Geometry check sheet. Reference: the model listing, model coordinates, mm. A direction names the side the tool comes from. Coordinates: 2 decimals unless noted, no trailing zeros. Write each loop counter-clockwise with the first axis right and the second up, starting at its lowest first coordinate (ties: lowest second). Pieces come first, ordered by that corner, then holes. Notation, with made-up numbers: (61, 69) -> (101, 69) arc R18 cw to (101, 91) -> close; hole circle Ø9 at (78, 36.25). An arc over 180 degrees is marked (long way). Answer in a Markdown table with one row per item. Add a question column.
Q1. Section check D-D, the plane x = -15. Record the boundary of the cut face in (y, z).
Q2. Section check B-B, the plane x = 53.5. Record the boundary of the cut face in (y, z), and give its area (3 significant figures).
Q3. Tool access check on faces 1 (the face through (17.734, -76, -7)), 2 (the face through (-31, -56.815, 23)), 3 (the face through (35, -32, -27.231)), 4 (the face through (-35, -14, 27.231)), 5 (the face through (-36, -42, -17.718)). Record the directions out of +Z, -Z, +X, -X, +Y, -Y that give a thin tool (end or side, any length) a straight path to the whole face; none if there is none.
Q4. Release check for a two-part mould opening along X. For faces 6 (the face through (-35, -70, 27.231)), 7 (the face through (10.484, -48.74, -9.389)), 8 (the face through (-71.588, -42, 5)) record: pulls with the +X half, pulls with the -X half, needs draft (parallel to the pull), parting line crosses it, or undercut.
Q5. Section check A-A, the plane y = -79. Record the boundary of the cut face in (x, z), and give its area (3 significant figures).
Q6. Gauge pin test, flat ends, axial feed: P1, Ø4, axis at x = 42, y = -44.5, coming from the +Z side; P2, Ø15.5, axis at x = 52.64, y = -18.85, coming from the +Z side; P3, Ø12.5, axis at x = 52.64, y = -48.42, coming from the -Z side; P4, Ø17, axis at x = 17.73, y = -18.85, coming from the +Z side. Record the tip position at first contact, or that the pin passes through.
Q7. Section check C-C, the plane z = 0.5. Record the boundary of the cut face in (x, y), and give its area (3 significant figures).
Q8. Thickness scan on line 1 (Y direction, x = 52.5, z = -16); line 2 (Y direction, x = -37, z = 22); line 3 (X direction, y = -18.5, z = -15.5). Record the ranges inside material, lowest first.
```python
from build123d import *

# Parameters (mm, degrees)
F1_DEPTH = 67.056
F2_W     = 71.5878978372
F2_H     = 5.1953196526
F3_DEPTH = 186.436
F4_DEPTH = 17.272
F5_DEPTH = 4.318
F6_W     = 29.3028312416
F6_H     = 7.5802523643
F7_DEPTH = 176.784
F8_R     = 7.2573235492
F8_R_2   = 6.8780266073
F8_R_3   = 6.6715099214
F8_R_4   = 6.5534755611
F9_DEPTH = 94.742


with BuildPart() as f1:
    # F0 (on Front) → F1 (new body)
    with BuildSketch(Plane.XZ):
        Polygon((71.5878978372, -27.2314734757), (0, 27.2314734757), (-71.5878978372, 27.2314734757), (-71.5878978372, -27.2314734757), align=None)
    extrude(amount=F1_DEPTH)

    # F2 (on face) → F3 (cut)
    with BuildSketch(Plane.XZ.offset(67.056)):
        with Locations((-35.7939489186, -24.6338136494)):
            Rectangle(F2_W, F2_H)
    extrude(amount=-F3_DEPTH, mode=Mode.SUBTRACT)

    # F2 (on face) → F4 (join)
    with BuildSketch(Plane.XZ.offset(67.056)):
        Polygon((17.7344851975, -27.2314734757), (17.7344851975, 13.739356013), (0, 27.2314734757), (-71.5878978372, 27.2314734757), (-71.5878978372, -22.0361538231), (0, -22.0361538231), (0, -27.2314734757), align=None)
    extrude(amount=F4_DEPTH)

    # F5 (cut): a face of the model
    f5_faces = [f1.faces().sort_by_distance(p)[0] for p in [
        (-35.7939489186, -42.164, -22.0361538231),
    ]]
    extrude(f5_faces, amount=-F5_DEPTH, mode=Mode.SUBTRACT)

    # F6 (on face) → F7 (cut)
    with BuildSketch(Plane(origin=(-71.5878978372, 0, 0), x_dir=(0, -1, 0), z_dir=(-1, 0, 0))):
        with Locations((42.164, 23.4413472936)):
            Rectangle(F6_W, F6_H)
    extrude(amount=-F7_DEPTH, mode=Mode.SUBTRACT)

    # F8 (on face) → F9 (cut)
    with BuildSketch(Plane(origin=(0, 0, -27.2314734757), x_dir=(1, 0, 0), z_dir=(0, 0, -1))):
        with Locations((17.7344851975, 48.4204255044)):
            Circle(F8_R)
        with Locations((52.6362881064, 48.4204255044)):
            Circle(F8_R_2)
        with Locations((52.6362881064, 18.8494753093)):
            Circle(F8_R_3)
        with Locations((17.7344851975, 18.8494753093)):
            Circle(F8_R_4)
    extrude(amount=-F9_DEPTH, mode=Mode.SUBTRACT)


solid = f1.part
```
Calculated:
| question | item | result |
|---|---|---|
| 1 | outline | (-84.33, -17.72) -> (0, -17.72) -> (0, 27.23) -> (-27.51, 27.23) -> (-27.51, 19.65) -> (-56.82, 19.65) -> (-56.82, 27.23) -> (-84.33, 27.23) -> close |
| 2 | outline | (-67.06, -27.23) -> (-55.24, -27.23) -> (-55.24, -13.47) -> (-67.06, -13.47) -> close; (-41.6, -27.23) -> (-25.46, -27.23) -> (-25.46, -13.47) -> (-41.6, -13.47) -> close; (-12.23, -27.23) -> (0, -27.23) -> (0, -13.47) -> (-12.23, -13.47) -> close |
| 2 | area | 553 mm² |
| 3 | face 1 | +Z, -Z, +X, -Y |
| 3 | face 2 | +Z, +X, -X |
| 3 | face 3 | -Z, +X, -X, +Y, -Y |
| 3 | face 4 | +Z, +X, -X, +Y, -Y |
| 3 | face 5 | -Z, -X, +Y, -Y |
| 4 | face 6 | needs draft |
| 4 | face 7 | undercut |
| 4 | face 8 | pulls with the -X half |
| 5 | outline | (-71.59, -17.72) -> (0, -17.72) -> (0, -27.23) -> (17.73, -27.23) -> (17.73, 13.74) -> (0, 27.23) -> (-71.59, 27.23) -> close |
| 5 | area | 4,060 mm² |
| 6 | P1 | stops at z = -3.2 |
| 6 | P2 | stops at z = -6.92 |
| 6 | P3 | passes through |
| 6 | P4 | stops at z = 20.21 |
| 7 | outline | (-71.59, -84.33) -> (17.73, -84.33) -> (17.73, -67.06) -> (35.14, -67.06) -> (35.14, 0) -> (-71.59, 0) -> close; hole circle Ø14.51 at (17.73, -48.42); hole circle Ø13.11 at (17.73, -18.85) |
| 7 | area | 8,400 mm² |
| 8 | line 1 | y = -67.06 to -55.3, -41.54 to -25.52, -12.18 to 0 |
| 8 | line 2 | y = -84.33 to -56.82, -27.51 to 0 |
| 8 | line 3 | x = -71.59 to 11.19, 24.28 to 45.97 |
